```python
from build123d import *

# Parameters (mm, degrees)
ESQUISSE1_R        = 25
ESQUISSE1_R_2      = 23
ESQUISSE1_R_3      = 3
ESQUISSE1_R_4      = 1.5
BOSS_EXTRU_1_DEPTH = 5
CONG_1_R           = 50
CONG_2_R           = 50


with BuildPart() as part:
    # Esquisse1 → Boss.-Extru.1 (new body)
    # profile 1 of 5: a face of its own
    with BuildSketch(Plane.XY):
        Circle(ESQUISSE1_R)
        Circle(ESQUISSE1_R_2, mode=Mode.SUBTRACT)
    # profile 2 of 5: a face of its own
    with BuildSketch(Plane.XY):
        with BuildLine():
            Line((30, 3), (22.547920633, 10.797743982))
            ThreePointArc((22.547920633, 10.797743982), (24.379274147, 5.536333812), (25, 0))
            ThreePointArc((25, 0), (24.379274147, -5.536333812), (22.547920633, -10.797743982))
            Line((22.547920633, -10.797743982), (30, -3))
            ThreePointArc((30, -3), (27, 0), (30, 3))
        make_face()
    # profile 3 of 5: a face of its own
    with BuildSketch(Plane.XY):
        with Locations((30, 0)):
            Circle(ESQUISSE1_R_3)
        with Locations((30, 0)):
            Circle(ESQUISSE1_R_4, mode=Mode.SUBTRACT)
    # profile 4 of 5: a face of its own
    with BuildSketch(Plane.XY):
        with Locations((-30, 0)):
            Circle(ESQUISSE1_R_3)
        with Locations((-30, 0)):
            Circle(ESQUISSE1_R_4, mode=Mode.SUBTRACT)
    # profile 5 of 5: a face of its own
    with BuildSketch(Plane.XY):
        with BuildLine():
            Line((-22.547920633, 10.797743982), (-30, 3))
            ThreePointArc((-30, 3), (-27.878679656, 2.121320344), (-27, 0))
            ThreePointArc((-27, 0), (-27.878679656, -2.121320344), (-30, -3))
            Line((-30, -3), (-22.547920633, -10.797743982))
            ThreePointArc((-22.547920633, -10.797743982), (-25, 0), (-22.547920633, 10.797743982))
        make_face()
    extrude(amount=BOSS_EXTRU_1_DEPTH)

    # Congé1
    cong_1_edges = [part.edges().sort_by_distance(p)[0] for p in [
        (22.547920633, -10.797743982, 2.5),
        (-22.547920633, -10.797743982, 2.5),
        (-22.547920633, 10.797743982, 2.5),
        (22.547920633, 10.797743982, 2.5),
    ]]
    fillet(cong_1_edges, radius=CONG_1_R)

    # Congé2
    # the kernel refuses this fillet: 50 mm, written as the material it adds along each edge
    with BuildSketch(Plane(origin=(-30, 3, 0), x_dir=(0.690901472787751, 0.722948929662197, 0), z_dir=(0, 0, 1))) as cong_2_piece_1:
        with BuildLine():
            CenterArc((8.249869656, 49.8931531), CONG_2_R, 258.662988377, 7.590639101)
            Line((-1.579108122, 0.868759215), (-1.775687678, -0.111728663))
            ThreePointArc((-1.775687678, -0.111728663), (-1.20479652, -0.320389641), (-0.72294893, -0.690901473))
            Line((-0.72294893, -0.690901473), (0, -1))
            ThreePointArc((0, -1), (2.491435997, -1), (4.917532041, -0.997863062))
            Line((4.917532041, -0.997863062), (4.982871995, 0))
        make_face()
    extrude(amount=5)
    with BuildSketch(Plane(origin=(-30, -3, 0), x_dir=(-0.9538179852697427, 0.30038517103207485, 0), z_dir=(0, 0, 1))) as cong_2_piece_2:
        with BuildLine():
            CenterArc((16.821569578, 47.690899263), CONG_2_R, 244.928622049, 7.590639101)
            Line((-4.365780115, 2.401869543), (-4.789527109, 1.496088949))
            ThreePointArc((-4.789527109, 1.496088949), (-2.664915192, 0.324777383), (-0.482025134, -0.876157389))
            Line((-0.482025134, -0.876157389), (0.300385171, -0.953817985))
            ThreePointArc((0.300385171, -0.953817985), (0.901155513, -0.861453956), (1.501925855, -0.953817985))
            Line((1.501925855, -0.953817985), (1.802311026, 0))
        make_face()
    extrude(amount=5)
    with BuildSketch(Plane(origin=(30, -3, 0), x_dir=(0.9538179852697404, 0.30038517103208245, 0), z_dir=(0, 0, 1))) as cong_2_piece_3:
        with BuildLine():
            CenterArc((16.821569578, -47.690899263), CONG_2_R, 107.48073885, 7.590639101)
            Line((-4.365780115, -2.401869543), (-4.789527109, -1.496088949))
            ThreePointArc((-4.789527109, -1.496088949), (-2.664915192, -0.324777383), (-0.482025134, 0.876157389))
            Line((-0.482025134, 0.876157389), (0.300385171, 0.953817985))
            ThreePointArc((0.300385171, 0.953817985), (0.901155513, 0.861453956), (1.501925855, 0.953817985))
            Line((1.501925855, 0.953817985), (1.802311026, 0))
        make_face()
    extrude(amount=5)
    with BuildSketch(Plane(origin=(30, 3, 0), x_dir=(-0.6909014727877525, 0.7229489296621958, 0), z_dir=(0, 0, 1))) as cong_2_piece_4:
        with BuildLine():
            CenterArc((8.249869656, -49.8931531), CONG_2_R, 93.746372522, 7.590639101)
            Line((-1.579108122, -0.868759215), (-1.775687678, 0.111728663))
            ThreePointArc((-1.775687678, 0.111728663), (-1.20479652, 0.320389641), (-0.72294893, 0.690901473))
            Line((-0.72294893, 0.690901473), (0, 1))
            ThreePointArc((0, 1), (2.491435997, 1), (4.917532041, 0.997863062))
            Line((4.917532041, 0.997863062), (4.982871995, 0))
        make_face()
    extrude(amount=5)


solid = part.part
```
Check sheet for the modelled part. Datum: model origin and axes. Units: mm. Coordinates: 2 decimals unless noted, no trailing zeros. Order: outer loops, then holes, each group sorted by start corner. A loop starts at its lowest first (then second) coordinate and runs counter-clockwise, first axis right, second up. Notation, with made-up numbers: M -21,-30 L 27,-30 A25 cw 27,0 Z; hole C 32,28.5 d10. An arc over 180 degrees is marked long. Write each question's results on one line, items separated by ' | '. Start each with the question number.
1. Cross-section at B-B on y = 16. Record the cut outline in (x, z), and give its area (3 significant figures).
2. Material ranges on probe 1 along Y at (x, z) = (0, 1.35); probe 2 along X at (y, z) = (-13.5, 1.95); probe 3 along Y at (x, z) = (-17, 3.5), recorded low to high.
3. Cross-section at D-D on y = 0. Record the cut outline in (x, z).
4. Cross-section at A-A on x = 0. Record the cut outline in (y, z), and give its area (3 significant figures).
5. Go/stop test with flat-tipped pins: P1, Ø2, axis at y = 5.5, z = 1.5, coming from the +X side; P2, Ø1.8, axis at x = -30, y = 0, coming from the +Z side; P3, Ø4, axis at x = 30, y = 0, coming from the +Z side; P4, Ø2, axis at y = -17.5, z = 3, coming from the -X side. Record where each tip stops, or that it passes through.
6. Cross-section at C-C on z = 0.75. Record the cut outline in (x, y), and give its area (3 significant figures).
7. Mould release check, pull along X, two halves, no side actions. Record for faces 1 (the face through (-23.61, 9.98, 2.54)), 2 (the face through (21, 10, 0)), 3 (the face through (28.5, 0.07, 2.46)): +X half, -X half, draft (parallel to the pull), parting line (faces both ways), or undercut.
Checks:
1) outline: M -19.21,0 L -16.52,0 L -16.52,5 L -19.21,5 Z; M 16.52,0 L 19.21,0 L 19.21,5 L 16.52,5 Z | area: 26.9 mm²
2) probe 1: y = -25 to -23, 23 to 25 | probe 2: x = -21.04 to -18.62, 18.62 to 21.04 | probe 3: y = -18.33 to -15.49, 15.49 to 18.33
3) outline: M -33,0 L -31.5,0 L -31.5,5 L -33,5 Z; M -28.5,0 L -23,0 L -23,5 L -28.5,5 Z; M 23,0 L 28.5,0 L 28.5,5 L 23,5 Z; M 31.5,0 L 33,0 L 33,5 L 31.5,5 Z
4) outline: M -25,0 L -23,0 L -23,5 L -25,5 Z; M 23,0 L 25,0 L 25,5 L 23,5 Z | area: 20.0 mm²
5) P1: stops at x = 29 | P2: passes through | P3: stops at z = 5 | P4: stops at x = -18.78
6) outline: M -31.72,-2.46 A50 cw -26.56,-6.6 A50 cw -20.9,-13.72 A25 ccw 20.9,-13.72 A50 cw 26.56,-6.6 A50 cw 31.72,-2.46 A3 ccw 31.72,2.46 A50 cw 26.56,6.6 A50 cw 20.9,13.72 A25 ccw -20.9,13.72 A50 cw -26.56,6.6 A50 cw -31.72,2.46 A3 ccw Z; hole C -30,0 d3; hole C 0,0 d46; hole C 30,0 d3 | area: 460 mm²
7) face 1: -X half | face 2: draft | face 3: undercut
